Can you work these out from the model? Positions are in its coordinate system, mm. Face numbers are marked on the shaded views. A direction names the side the tool comes from. Round coordinates to 2 decimals unless told otherwise and drop trailing zeros. Loops run counter-clockwise (first coordinate to the right, second up) from the corner with the lowest first, then second, coordinate; pieces in that order, holes last. Notation, with made-up numbers: (27.5, 69.25) -> (81.5, 69.25) arc R27 cw to (81.5, 99.25) -> close; hole circle Ø2 at (12.25, 47). An arc over 180 degrees is marked (long way). Use a Markdown table: item, result.
from build123d import *

# Parameters (mm, degrees)
F0_W     = 45.72
F0_H     = 133.35
F1_DEPTH = 2.54
F2_R     = 1.5875
F3_DEPTH = 136.525
F4_DEPTH = 3.175
F5_R     = 1.5875
F7_DEPTH = 25.4
F9_DEPTH = 25.4


with BuildPart() as f1:
    # F0 (on Top) → F1 (new body)
    with BuildSketch(Plane.XY):
        Rectangle(F0_W, F0_H)
    extrude(amount=F1_DEPTH)

    # F2 (on face) → F3 (join)
    with BuildSketch(Plane.XZ.offset(66.675)):
        with Locations((22.86, 2.54)):
            Circle(F2_R)
    extrude(amount=-F3_DEPTH)

    # F2 (on face) → F4 (join)
    with BuildSketch(Plane.XZ.offset(66.675)):
        with Locations((22.86, 2.54)):
            Circle(F2_R)
    extrude(amount=F4_DEPTH)

    # F5
    f5_edges = [f1.edges().sort_by_distance(p)[0] for p in [
        (21.2725, -69.85, 2.54),
        (21.2725, 69.85, 2.54),
    ]]
    fillet(f5_edges, radius=F5_R)

    # F6 (on face) → F7 (cut)
    with BuildSketch(Plane(origin=(0, 0, 0), x_dir=(1, 0, 0), z_dir=(0, 0, -1))):
        with BuildLine():
            ThreePointArc((-17.907, 0), (-16.51, -1.397), (-15.113, 0))
            ThreePointArc((-15.113, 0), (-16.51, 1.397), (-17.907, 0))
        make_face()
    extrude(amount=-F7_DEPTH, mode=Mode.SUBTRACT)

    # F8 (on face) → F9 (cut)
    with BuildSketch(Plane(origin=(0, 0, 0), x_dir=(1, 0, 0), z_dir=(0, 0, -1))):
        Polygon((8.20166, 46.397122), (0, 56.093656), (-8.20166, 46.397122), (0, 22.357721), align=None)
        Polygon((-8.20166, -46.310099), (0, -56.006633), (8.20166, -46.310099), (0, -22.270698), align=None)
        Polygon((-6.35, -3.517313), (0, -14.515836), (6.35, -3.517313), align=None)
        Polygon((6.35, 3.899692), (0, 14.898214), (-6.35, 3.899692), align=None)
    extrude(amount=-F9_DEPTH, mode=Mode.SUBTRACT)


solid = f1.part
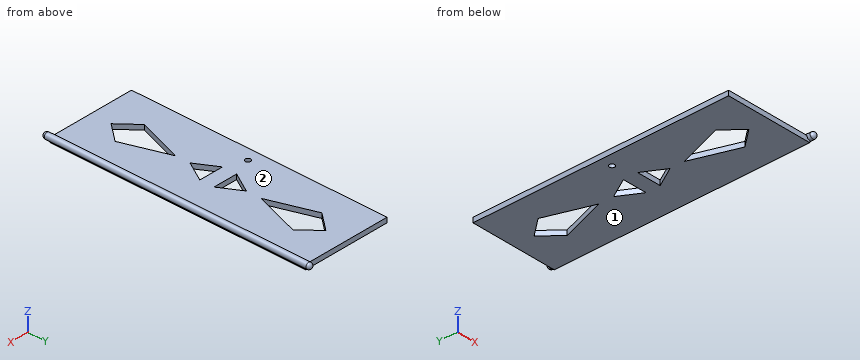
1. I want a section at A-A (y = 0). Please give me the cut outline in (x, z) (1 decimal), plus the area to 3 significant figures.
Answer sheet:
| item | result |
|---|---|
| outline | (-22.9, 0) -> (-17.9, 0) -> (-17.9, 2.5) -> (-22.9, 2.5) -> close; (-15.1, 0) -> (22.9, 0) -> (22.9, 1) arc R1.6 ccw (long way) to (21.3, 2.5) -> (-15.1, 2.5) -> close |
| area | 115 mm² |
2. I want a section at C-C (z = 1.8). State how many separate pieces and enclosed holes the cut face has, plus the area to 3 significant figures.
Answer sheet:
| item | result |
|---|---|
| separate pieces | 1 |
| enclosed holes | 5 |
| area | 5,600 mm² |
3. I want a section at B-B (x = -16.51). Please give me the cut outline in (y, z) (3 decimals), plus the area to 3 significant figures.
Answer sheet:
| item | result |
|---|---|
| outline | (-66.675, 0) -> (-1.397, 0) -> (-1.397, 2.54) -> (-66.675, 2.54) -> close; (1.397, 0) -> (66.675, 0) -> (66.675, 2.54) -> (1.397, 2.54) -> close |
| area | 332 mm² |
4. Which directions (+Z, -Z, +X, -X, +Y, -Y) give clear straight access to the entire face, cutting with the end or side of a thin tool? Please do the marked faces 1 and 2.
Answer sheet:
| item | result |
|---|---|
| face 1 | -Z, +X, -X, +Y, -Y |
| face 2 | +Z, -X, +Y, -Y |
5. I want a section at D-D (y = -26). Please give me the cut outline in (x, z) (1 decimal), plus the area to 3 significant figures.
Answer sheet:
| item | result |
|---|---|
| outline | (-22.9, 0) -> (-1.2, 0) -> (-1.2, 2.5) -> (-22.9, 2.5) -> close; (1.2, 0) -> (22.9, 0) -> (22.9, 1) arc R1.6 ccw (long way) to (21.3, 2.5) -> (1.2, 2.5) -> close |
| area | 116 mm² |
6. I need wall thicknesses on line 1 (Y direction, x = -16.51, z = 1.9) (3 decimals); line 2 (Z direction, x = 17, y = 49); line 3 (X direction, y = -8.5, z = 2.3). Which ranges of each line are inside material? Lowest first, please.
Answer sheet:
| item | result |
|---|---|
| line 1 | y = -66.675 to -1.397, 1.397 to 66.675 |
| line 2 | z = 0 to 2.54 |
| line 3 | x = -22.86 to -3.69, 3.69 to 24.43 |
7. Will these pins go through, and if not, where does the flat tip stop? pin 1 Ø10 at (x, y) = (16.5, -20) entering from +Z; pin 2 Ø1.3 at (x, z) = (-3, 1) entering from +Y (3 decimals); pin 3 Ø3.5 at (x, y) = (-16.51, 0) entering from +Z.
Answer sheet:
| item | result |
|---|---|
| pin 1 | stops at z = 3.36 |
| pin 2 | stops at y = 66.675 |
| pin 3 | stops at z = 2.54 |
